Part print with two shaded views. Sizes in mm from the minimum x, y, z corner. Round coordinates to 2 decimals unless told otherwise and drop trailing zeros. Write each loop counter-clockwise with the first axis right and the second up, starting at its lowest first coordinate (ties: lowest second). Pieces come first, ordered by that corner, then holes. Notation, with made-up numbers: (-35, -15) -> (-16, -15) arc R27 cw to (-16, 2) -> close; hole circle Ø3 at (57.5, -8.5). An arc over 180 degrees is marked (long way). Put each result on its own line as item: value. Start each with the question number.
1. Pull direction Y, two halves, no side cores. Call the marked faces 1, 2, 3 and 4: pulls with the +Y half, pulls with the -Y half, needs draft (parallel to the pull), parting line crosses it, or undercut.
2. Saw through at A-A on y = 21. List the corners of the cut face in (x, z), and give its area (3 significant figures).
3. Saw through at C-C on z = 2.5. List the corners of the cut face in (x, y).
4. Flat gauge pin, fed straight in: P1, Ø3, axis at x = 15, y = 12.5, coming from the +Z side. Where does the tip first touch, or does it go through?
5. Saw through at B-B on x = 15.75. List the corners of the cut face in (y, z), and give its area (3 significant figures).
6. Drill centre lines: line 1 (X direction, y = 16.25, z = 6.75); line 2 (Y direction, x = 10.25, z = 4.25) (1 decimal); line 3 (X direction, y = 18, z = 7.75). Where is each one in solid material? Low to high. Write a range as from..to.
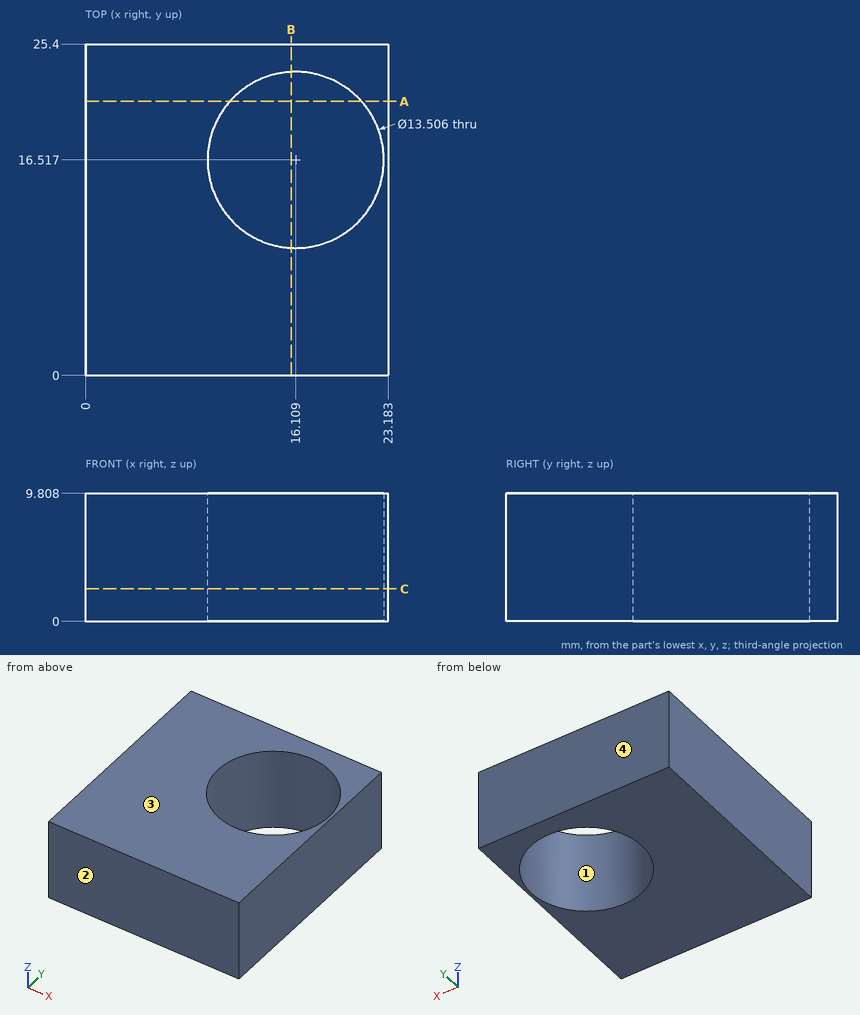
Return value:
1. face 1: undercut
1. face 2: pulls with the -Y half
1. face 3: needs draft
1. face 4: pulls with the +Y half
2. outline: (0, 0) -> (11.06, 0) -> (11.06, 9.81) -> (0, 9.81) -> close; (21.16, 0) -> (23.18, 0) -> (23.18, 9.81) -> (21.16, 9.81) -> close
2. area: 128 mm^2
3. outline: (0, 0) -> (23.18, 0) -> (23.18, 25.4) -> (0, 25.4) -> close; hole circle Ø13.51 at (16.11, 16.52)
4. P1: passes through
5. outline: (0, 0) -> (9.77, 0) -> (9.77, 9.81) -> (0, 9.81) -> close; (23.26, 0) -> (25.4, 0) -> (25.4, 9.81) -> (23.26, 9.81) -> close
5. area: 117 mm^2
6. line 1: x = 0..9.36, 22.86..23.18
6. line 2: y = 0..13.2, 19.9..25.4
6. line 3: x = 0..9.52, 22.7..23.18
